```python
from build123d import *

# Parameters (mm, degrees)
SKETCH2_R               = 49
SKETCH2_R_2             = 46
BOSS_EXTRUDE1_DEPTH     = 120
SKETCH5_R               = 1.5
CUT_EXTRUDE2_DEPTH      = 50
CUT_EXTRUDE2_DEPTH_BACK = 50
SKETCH6_R               = 1.5
CUT_EXTRUDE3_DEPTH      = 50.0000001
CUT_EXTRUDE3_DEPTH_BACK = 50.000000102


with BuildPart() as part:
    # Sketch2 → Boss-Extrude1 (new body)
    with BuildSketch(Plane(origin=(0, 0, 0), x_dir=(1, 0, 0), z_dir=(0, 1, 0))):
        Circle(SKETCH2_R)
        Circle(SKETCH2_R_2, mode=Mode.SUBTRACT)
    extrude(amount=BOSS_EXTRUDE1_DEPTH)

    # Sketch5 → Cut-Extrude2 (cut, two sides)
    with BuildSketch(Plane(origin=(0, 0, 0), x_dir=(0, 0, -1), z_dir=(1, 0, 0))) as cut_extrude2_sk:
        with Locations((0, 108.5)):
            Circle(SKETCH5_R)
    extrude(amount=CUT_EXTRUDE2_DEPTH, mode=Mode.SUBTRACT)
    extrude(cut_extrude2_sk.sketch, amount=-CUT_EXTRUDE2_DEPTH_BACK, mode=Mode.SUBTRACT)

    # Sketch6 → Cut-Extrude3 (cut, two sides)
    with BuildSketch(Plane(origin=(0, 0, 0), x_dir=(0, 0, -1), z_dir=(1, 0, 0))) as cut_extrude3_sk:
        with Locations((0, 15)):
            Circle(SKETCH6_R)
        with Locations((0, 43)):
            Circle(SKETCH6_R)
    extrude(amount=CUT_EXTRUDE3_DEPTH, mode=Mode.SUBTRACT)
    extrude(cut_extrude3_sk.sketch, amount=-CUT_EXTRUDE3_DEPTH_BACK, mode=Mode.SUBTRACT)


solid = part.part
```
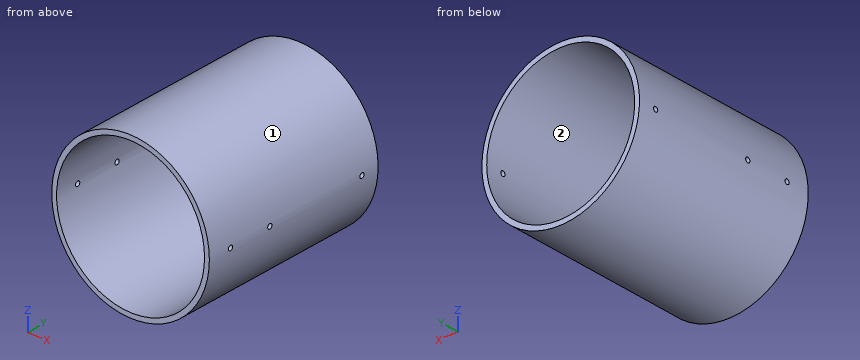
Work out the finished part from the listing and answer in its coordinate system (mm). Face numbers are marked on the shaded views. Give positions to 0.01 mm unless a question says otherwise; leave off trailing zeros. Loops run counter-clockwise (first coordinate to the right, second up) from the corner with the lowest first, then second, coordinate; pieces in that order, holes last. Notation, with made-up numbers: (85.25, -25) -> (124.25, -25) arc R13 ccw to (124.25, -1) -> close; hole circle Ø6 at (83.5, 83.25). An arc over 180 degrees is marked (long way). Write item = value, one per line. Start each with the question number.
(1) The mould has two halves that part along Z. Classify the marked faces 1 and 2: +Z half, -Z half, draft (parallel to the pull), parting line (faces both ways), or undercut.
(2) Find section C-C on z = 0. Give the number of separate pieces and of enclosed holes in the cut face, and give its area (3 significant figures).
(3) Find section D-D on y = 70. Give the vertices of the cut face in (x, z), and give its area (3 significant figures).
(4) Given pin 1 Ø1 at (y, z) = (21, -24.5) entering from +X; pin 2 Ø2.5 at (y, z) = (15, 0) entering from +X; pin 3 Ø6 at (x, y) = (-12.5, 23.5) entering from +Z; pin 4 Ø12 at (x, y) = (-20, 61) entering from +Z, each flat-ended and moving along its own axis, determine where each tip first touches the part or whether it passes through.
(5) Find section A-A on x = 0. Give the vertices of the cut face in (y, z), and give its area (3 significant figures).
(6) Find section B-B on z = 41.5. Give the vertices of the cut face in (x, y).
(7) Find the intervals of material crossed by probe 1 along Y at (x, z) = (-48.3, 0); probe 2 along Z at (x, y) = (-0.5, 29.5); probe 3 along Z at (x, y) = (-23.5, 21), in increasing order. Write a range as from..to.
From the geometry:
q1.face_1 = parting line
q1.face_2 = undercut
q2.separate_pieces = 8
q2.enclosed_holes = 0
q2.area = 666 mm^2
q3.outline = circle Ø98 at (0, 0); hole circle Ø92 at (0, 0)
q3.area = 895 mm^2
q4.pin_1 = 42.72
q4.pin_2 = through
q4.pin_3 = 48.07
q4.pin_4 = 46.96
q5.outline = (0, -49) -> (120, -49) -> (120, -46) -> (0, -46) -> close; (0, 46) -> (120, 46) -> (120, 49) -> (0, 49) -> close
q5.area = 720 mm^2
q6.outline = (-26.05, 0) -> (-19.84, 0) -> (-19.84, 120) -> (-26.05, 120) -> close; (19.84, 0) -> (26.05, 0) -> (26.05, 120) -> (19.84, 120) -> close
q7.probe_1 = 0..13.5, 16.5..41.5, 44.5..107, 110..120
q7.probe_2 = -49..-46, 46..49
q7.probe_3 = -43..-39.54, 39.54..43
